```python
from build123d import *

# Parameters (mm, degrees)
SKETCH3_W           = 70
SKETCH3_H           = 60
BOSS_EXTRUDE1_DEPTH = 30
SKETCH4_W           = 6
SKETCH4_H           = 20
CUT_EXTRUDE1_DEPTH  = 82.853527719


with BuildPart() as part:
    # Sketch3 → Boss-Extrude1 (new body)
    with BuildSketch(Plane(origin=(0, 0, 0), x_dir=(1, 0, 0), z_dir=(0, 1, 0))):
        Rectangle(SKETCH3_W, SKETCH3_H)
    extrude(amount=-BOSS_EXTRUDE1_DEPTH)

    # Sketch4 → Cut-Extrude1 (cut, through all)
    with BuildSketch(Plane(origin=(35, 0, 0), x_dir=(0, 0, -1), z_dir=(1, 0, 0))):
        with Locations((-15, 0)):
            Rectangle(SKETCH4_W, SKETCH4_H)
    cut_extrude1 = extrude(amount=-CUT_EXTRUDE1_DEPTH, mode=Mode.SUBTRACT)

    # Mirror1: Cut-Extrude1 across plane
    add(cut_extrude1.mirror(Plane.XY), mode=Mode.SUBTRACT)


solid = part.part
```
The model under review builds one solid part; all positions refer to its coordinate system, in mm. A direction names the side the tool comes from. Give positions to 0.01 mm unless a question says otherwise; leave off trailing zeros. Write each loop counter-clockwise with the first axis right and the second up, starting at its lowest first coordinate (ties: lowest second). Pieces come first, ordered by that corner, then holes. Notation, with made-up numbers: (63.25, -29) - (110.25, -29) arc R28 cw to (110.25, -2) - close; hole circle Ø9 at (48.25, 78.25). An arc over 180 degrees is marked (long way). Answer in a Markdown table with one row per item. Add a question column.
1. Wall thickness on line 1 along Z through (x, y) = (22, -4.5); line 2 along Y through (x, z) = (-23, 14.5): over which ranges is each line inside the solid? List them lowest first. Write a range as [from, to].
2. We need section B-B on x = 3.5. Write out the cut boundary in (y, z).
3. Tool access review of faces 1 (the flat face through (-35, -15, 0)), 2 (the flat face through (0, -5, -18)): name each direction out of +Z, -Z, +X, -X, +Y, -Y from which nothing blocks a thin tool from reaching the whole face with its end or side.
4. Insertion check: P1, Ø1, axis at x = -6, z = 21.5, coming from the +Y side; P2, Ø1.8, axis at x = -8.5, z = -15.5, coming from the +Y side. Each pin has a flat end and moves straight along its axis. Give the tip position at first contact, or say it passes through.
5. Draft analysis for pull direction Z (two halves, no side actions). For faces 3 (the flat face through (0, -5, 12)), 4 (the flat face through (0, -30, 0)), 5 (the flat face through (0, -15, -30)), state which applies: +Z half, -Z half, draft (parallel to the pull), parting line (faces both ways), or undercut.
6. We need section C-C on z = 14.5. Write out the cut boundary in (x, y), then the cut area to 3 significant figures.
7. We need section A-A on y = -5.75. Write out the cut boundary in (x, z).
Ans:
| question | item | result |
|---|---|---|
| 1 | line 1 | z = [-30, -18], [-12, 12], [18, 30] |
| 1 | line 2 | y = [-30, -10] |
| 2 | outline | (-30, -30) - (0, -30) - (0, -18) - (-10, -18) - (-10, -12) - (0, -12) - (0, 12) - (-10, 12) - (-10, 18) - (0, 18) - (0, 30) - (-30, 30) - close |
| 3 | face 1 | +Z, -Z, -X, +Y, -Y |
| 3 | face 2 | +X, -X, +Y |
| 4 | P1 | stops at y = 0 |
| 4 | P2 | stops at y = -10 |
| 5 | face 3 | undercut |
| 5 | face 4 | draft |
| 5 | face 5 | -Z half |
| 6 | outline | (-35, -30) - (35, -30) - (35, -10) - (-35, -10) - close |
| 6 | area | 1,400 mm^2 |
| 7 | outline | (-35, -30) - (35, -30) - (35, -18) - (-35, -18) - close; (-35, -12) - (35, -12) - (35, 12) - (-35, 12) - close; (-35, 18) - (35, 18) - (35, 30) - (-35, 30) - close |
